```python
from build123d import *

# Parameters (mm, degrees)
SKETCH1_R                               = 492.125
BOSS_EXTRUDE1_DEPTH                     = 3.175
F_3_8_CLEARANCE_HOLE1_D                 = 10.31748
F_1_4_CLEARANCE_HOLE_FOR_RFOF_D         = 7.14248
CIRPATTERN_18X_MOUNT_HOLES_IN_OUT_COUNT = 18


with BuildPart() as part:
    # Sketch1 → Boss-Extrude1 (new body)
    with BuildSketch(Plane(origin=(0, 0, 0), x_dir=(1, 0, 0), z_dir=(0, 1, 0))):
        Polygon((-715, 0), (-671.880223862, -244.544402478), (-547.72177683, -459.593140926), (-357.5, -619.208163706), (-124.158447032, -704.137543404), (124.158447032, -704.137543404), (357.5, -619.208163706), (547.72177683, -459.593140926), (671.880223862, -244.544402478), (715, 0), (671.880223862, 244.544402478), (547.72177683, 459.593140926), (357.5, 619.208163706), (124.158447032, 704.137543404), (-124.158447032, 704.137543404), (-357.5, 619.208163706), (-547.72177683, 459.593140926), (-671.880223862, 244.544402478), align=None)
        with Locations(Location((0, 0, 0), (0, 0, 270))):
            Circle(SKETCH1_R, mode=Mode.SUBTRACT)
    extrude(amount=BOSS_EXTRUDE1_DEPTH)

    # 3/8 Clearance Hole1 (through all)
    with Locations(Plane(origin=(0, 3.175, 0), x_dir=(1, 0, 0), z_dir=(0, 1, 0))):
        with Locations((-121.987844811, -691.827446491)):
            f_3_8_clearance_hole1 = Hole(F_3_8_CLEARANCE_HOLE1_D / 2)

    # 1/4 Clearance Hole for RFoF (through all)
    with Locations(Plane(origin=(0, 3.175, 0), x_dir=(1, 0, 0), z_dir=(0, 1, 0))):
        with Locations((-66.675, -499.905299908), (66.675, -499.905299908), (0, -499.905299908)):
            f_1_4_clearance_hole_for_rfof = Hole(F_1_4_CLEARANCE_HOLE_FOR_RFOF_D / 2)

    # CirPattern - 18x Mount Holes In_Out: 3/8 Clearance Hole1, 1/4 Clearance Hole for RFoF ×18 about axis
    cirpattern_18x_mount_holes_in_out_axis = Axis((0, 0, 0), (0, 1, 0))
    add([f_3_8_clearance_hole1.rotate(cirpattern_18x_mount_holes_in_out_axis, i * 360 / CIRPATTERN_18X_MOUNT_HOLES_IN_OUT_COUNT) for i in range(1, CIRPATTERN_18X_MOUNT_HOLES_IN_OUT_COUNT)], mode=Mode.SUBTRACT)
    add([f_1_4_clearance_hole_for_rfof.rotate(cirpattern_18x_mount_holes_in_out_axis, i * 360 / CIRPATTERN_18X_MOUNT_HOLES_IN_OUT_COUNT) for i in range(1, CIRPATTERN_18X_MOUNT_HOLES_IN_OUT_COUNT)], mode=Mode.SUBTRACT)


solid = part.part
```
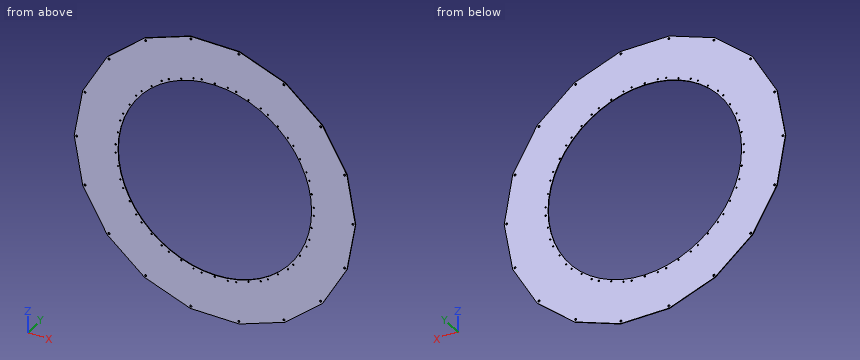
Work out the finished part from the listing and answer in its coordinate system (mm). Round coordinates to 2 decimals unless told otherwise and drop trailing zeros. Write each question's results on one line, items separated by ' | '. Start each with the question number.
1. Given pin 1 Ø9.5 at (x, z) = (0, -499.91) entering from +Y (3 decimals); pin 2 Ø1 at (y, z) = (2, 5.5) entering from -X; pin 3 Ø1.5 at (y, z) = (2.5, -141.5) entering from -X, each flat-ended and moving along its own axis, determine where each tip first touches the part or whether it passes through.
2. Find the intervals of material crossed by probe 1 along Z at (x, y) = (-234, 0.95); probe 2 along X at (y, z) = (2.1, 447); probe 3 along Z at (x, y) = (-493, 1.4), in increasing order. Write a range as from..to.
3. Section A-A (y = 0.8) is taken. State how many separate pieces and enclosed holes the cut face has, plus the area to 3 significant figures.
Evaluation:
1) pin 1: stops at y = 3.175 | pin 2: stops at x = -714.12 | pin 3: stops at x = -690.18
2) probe 1: z = -664.16..-450.51, -443.4..-432.93, 432.93..443.4, 450.51..664.16 | probe 2: x = -554.99..-540.56, -535.73..-237.2, -230.06..-205.86, 205.86..230.06, 237.2..535.73, 540.56..554.99 | probe 3: z = -505.51..-90.31, -83.3..83.3, 90.31..505.51
3) separate pieces: 1 | enclosed holes: 73 | area: 809,000 mm2
